```python
from build123d import *

# Parameters (mm, degrees)
SKETCH1_R           = 9.516746653
SKETCH1_R_2         = 4.309736146
EXTRUDE1_DEPTH      = 10
EXTRUDE1_DEPTH_BACK = 10
EXTRUDE2_DEPTH      = 25
EXTRUDE2_DEPTH_BACK = 10
EXTRUDE3_DEPTH      = 25


with BuildPart() as part:
    # Sketch1 → Extrude1 (new body, two sides)
    with BuildSketch(Plane.XY) as extrude1_sk:
        with Locations((-74.315769624, -7.949999587)):
            Circle(SKETCH1_R)
        with Locations((-74.315769624, -7.949999587)):
            Circle(SKETCH1_R_2, mode=Mode.SUBTRACT)
    extrude(amount=EXTRUDE1_DEPTH)
    extrude(extrude1_sk.sketch, amount=-EXTRUDE1_DEPTH_BACK)

    # Sketch2 → Extrude2 (add, two sides)
    with BuildSketch(Plane.XY.offset(10)) as extrude2_sk:
        with BuildLine():
            Line((-83.025654753, -11.784887838), (-106.019653855, -51.047339529))
            Line((-106.019653855, -51.047339529), (-106.019653855, -70.815363126))
            Line((-106.019653855, -70.815363126), (-44.938455036, -70.815363126))
            Line((-44.938455036, -70.815363126), (-69.620440041, -41.423398152))
            Line((-69.620440041, -41.423398152), (-69.620440041, -16.227822185))
            ThreePointArc((-69.620440041, -16.227822185), (-77.309777049, -16.983514208), (-83.025654753, -11.784887838))
        make_face()
    extrude(amount=EXTRUDE2_DEPTH)
    extrude(extrude2_sk.sketch, amount=-EXTRUDE2_DEPTH_BACK)

    # Sketch3 → Extrude3 (add)
    with BuildSketch(Plane.XY.offset(10)):
        with BuildLine():
            ThreePointArc((-83.025654753, -11.784887838), (-77.309777049, -16.983514208), (-69.620440041, -16.227822185))
            ThreePointArc((-69.620440041, -16.227822185), (-71.321762199, 1.083515033), (-83.025654753, -11.784887838))
        make_face()
    extrude(amount=EXTRUDE3_DEPTH)


solid = part.part
```
The listing builds one solid part. Answer for the finished solid, in the listing's coordinates (mm). A direction names the side the tool comes from. Coordinates: 2 decimals unless noted, no trailing zeros. Write each loop counter-clockwise with the first axis right and the second up, starting at its lowest first coordinate (ties: lowest second). Pieces come first, ordered by that corner, then holes. Notation, with made-up numbers: (14, 8) - (63, 8) arc R26 ccw to (63, 47) - close; hole circle Ø8 at (58.25, 58.25). An arc over 180 degrees is marked (long way). Return JSON: item names as keys, results as strings. Group by question number.
1. Determine the mould class of faces 1 (the flat face through (-76, -70.815, 18)), 2 (the flat face through (-106.02, -61, 18)), 3 (the flat face through (-69.62, -29, 18)) for opening direction Y: released by +Y, released by -Y, zero draft, split by the parting line, or undercut.
2. A cutting plane is placed at A-A, the plane z = 3. Determine the outline of the cut face in (x, y).
3. Which of the six approach directions +Z, -Z, +X, -X, +Y, -Y give full straight-line access (tool end or side, diameter ignored) to faces 4 (the flat face through (-74, -8, 10)), 5 (the flat face through (-83, -42, 35)), 6 (the flat face through (-57.107, -56.325, 17.745))?
4. A cutting plane is placed at D-D, the plane x = -52.5. Determine the outline of the cut face in (y, z).
5. Given pin 1 (3 mm diameter, centred on y = -47.5, z = 0, fed in from -X); pin 2 (3 mm diameter, centred on x = -93.5, z = 21, fed in from +Y); pin 3 (6 mm diameter, centred on x = -95.5, z = 25, fed in from +Y), each flat-ended and moving along its own axis, determine where each tip first touches the part or whether it passes through.
6. A cutting plane is placed at C-C, the plane z = 22.5. Determine the outline of the cut face in (x, y).
7. Straight lines are drawn through the part: L1, parallel to Z at x = -77, y = -24; L2, parallel to X at y = -7, z = -1; L3, parallel to Y at x = -93.5, z = 28. For each, find the intervals that lie inside material, in ascending order.
8. A cutting plane is placed at B-B, the plane y = -7.95. Determine the outline of the cut face in (x, z), plus the area to 3 significant figures.
Ans:
{
 "1": {"face 1": "released by -Y", "face 2": "zero draft", "face 3": "undercut"},
 "2": {"outline": "(-106.02, -70.82) - (-44.94, -70.82) - (-69.62, -41.42) - (-69.62, -16.23) arc R9.52 ccw (long way) to (-83.03, -11.78) - (-106.02, -51.05) - close; hole circle Ø8.62 at (-74.32, -7.95)"},
 "3": {"face 4": "-Z", "face 5": "+Z, +X, -X, +Y, -Y", "face 6": "+Z, -Z, +X"},
 "4": {"outline": "(-70.82, 0) - (-61.81, 0) - (-61.81, 35) - (-70.82, 35) - close"},
 "5": {"pin 1": "x = -104.82", "pin 2": "y = -27.11", "pin 3": "y = -27.96"},
 "6": {"outline": "(-106.02, -70.82) - (-44.94, -70.82) - (-69.62, -41.42) - (-69.62, -16.23) arc R9.52 ccw (long way) to (-83.03, -11.78) - (-106.02, -51.05) - close"},
 "7": {"L1": "0 to 35", "L2": "-83.78 to -78.52, -70.11 to -64.85", "L3": "-70.82 to -29.67"},
 "8": {"outline": "(-83.83, -10) - (-78.63, -10) - (-78.63, 10) - (-70.01, 10) - (-70.01, -10) - (-64.8, -10) - (-64.8, 35) - (-83.83, 35) - close", "area": "684 mm²"}
}
